from build123d import *

# Parameters (mm, degrees)
F0_R        = 37.5
F0_R_2      = 30.5
F1_DEPTH    = 40
F2_START    = 20
F0_R_3      = 12.5
F2_DEPTH    = 20
F3_START    = 39
F3_DEPTH    = 3
F4_S5_R     = 30.5
F4_T6_DEPTH = 47
F5_DEPTH    = 10


# Not quite as in the source:
# - a fillet or chamfer that OpenCascade refuses, or shapes differently, is made with other operations: its cross-section is extruded or revolved along the edge and cut away or added


with BuildPart() as f1:
    # F0 (on Top) → F1 (new body)
    with BuildSketch(Plane.XY):
        Circle(F0_R)
        Circle(F0_R_2, mode=Mode.SUBTRACT)
    extrude(amount=F1_DEPTH)

    # F0 (on Top) → F2 (join)
    with BuildSketch(Plane.XY.offset(F2_START)):
        Circle(F0_R_2)
        Circle(F0_R_3, mode=Mode.SUBTRACT)
    extrude(amount=F2_DEPTH)

    # F0 (on Top) → F3 (join)
    with BuildSketch(Plane.XY.offset(F3_START)):
        Circle(F0_R_3)
    extrude(amount=F3_DEPTH)

    # F4: chamfer of 19 on 1 edges, made by hand


with BuildPart() as f4_tool2:
    # F4_s3 → F4_t4 (revolve)
    with BuildSketch(Plane.XZ):
        Polygon((31.5, 20), (12.5, 39), (12.5, 20), align=None)
    revolve(axis=Axis((0, 0, 20), (0, 0, 1)))

    # F4_s5 → F4_t6 (intersect, symmetric)
    with BuildSketch(Plane.XY.offset(29.5)):
        Circle(F4_S5_R)
    extrude(amount=F4_T6_DEPTH, both=True, mode=Mode.INTERSECT)

    split(bisect_by=Plane.XY.offset(39), keep=Keep.BOTTOM)


with BuildPart() as f1_1:
    add(f1.part)

    # F4_t1: cut F4_tool2
    add(f4_tool2.part, mode=Mode.SUBTRACT)

    # F5 (cut): a face of the model
    f5_faces = [f1_1.faces().sort_by_distance(p)[0] for p in [
        (-36.4393398282, 0, 0),
    ]]
    extrude(f5_faces, amount=-F5_DEPTH, mode=Mode.SUBTRACT)


solid = f1_1.part
Geometry check sheet. Reference: the model listing, model coordinates, mm. A direction names the side the tool comes from. Give positions to 0.01 mm unless a question says otherwise; leave off trailing zeros. Loops run counter-clockwise (first coordinate to the right, second up) from the corner with the lowest first, then second, coordinate; pieces in that order, holes last. Notation, with made-up numbers: M -35,88.5 L -4,88.5 A26 ccw -4,112.5 Z; hole C 27,41.25 d10. An arc over 180 degrees is marked long. Answer as a JSON object with one key per item and string values. Group by question number.
Item 1: Sectioned sample at A-A on y = 0. Record the boundary of the cut face in (x, z).
Item 2: Access from +Z, -Z, +X, -X, +Y, -Y to the whole of each face (thin tool, end or side, straight path). Record for faces 4 (the flat face through (0, 0, 39)), 5 (the flat face through (0, 0, 42)), 6 (the flat face through (-9, 9, 40)).
Item 3: Sectioned sample at C-C on z = 16.5. Record the boundary of the cut face in (x, y).
Item 4: Mould release check, pull along Y, two halves, no side actions. Record for faces 1 (the flat face through (5.4, -30.4, 10)), 2 (the cylindrical face through (11.923, 3.755, 40.986)), 3 (the conical face through (12.756, 4.017, 38.126)): pulls with the +Y half, pulls with the -Y half, needs draft (parallel to the pull), parting line crosses it, or undercut.
Item 5: Material ranges on L1, parallel to Z at x = 12, y = 34; L2, parallel to Y at x = 0, z = 20.6; L3, parallel to Y at x = 10, z = 29.5, recorded low to high.
Item 6: Sectioned sample at D-D on z = 31.5. Record the boundary of the cut face in (x, y).
Item 7: Gauge pin test, flat ends, axial feed: pin 1 (1.5 mm diameter, centred on x = -15.5, z = 22.5, fed in from -Y); pin 2 (10 mm diameter, centred on x = -1, y = 27, fed in from +Z); pin 3 (2 mm diameter, centred on y = 17.5, z = 20, fed in from +X). Record the tip position at first contact, or that the pin passes through.
Findings below:
{
 "1": {"outline": "M -37.5,10 L -30.5,10 L -30.5,21 L -12.5,39 L 12.5,39 L 30.5,21 L 30.5,10 L 37.5,10 L 37.5,40 L 12.5,40 L 12.5,42 L -12.5,42 L -12.5,40 L -37.5,40 Z"},
 "2": {"face 4": "-Z", "face 5": "+Z, +X, -X, +Y, -Y", "face 6": "+Z"},
 "3": {"outline": "C 0,0 d75; hole C 0,0 d61"},
 "4": {"face 1": "needs draft", "face 2": "parting line crosses it", "face 3": "undercut"},
 "5": {"L1": "10 to 40", "L2": "-37.5 to -30.5, 30.5 to 37.5", "L3": "-36.14 to -19.6, 19.6 to 36.14"},
 "6": {"outline": "C 0,0 d75; hole C 0,0 d40"},
 "7": {"pin 1": "y = -34.48", "pin 2": "z = 40", "pin 3": "x = 33.67"}
}
